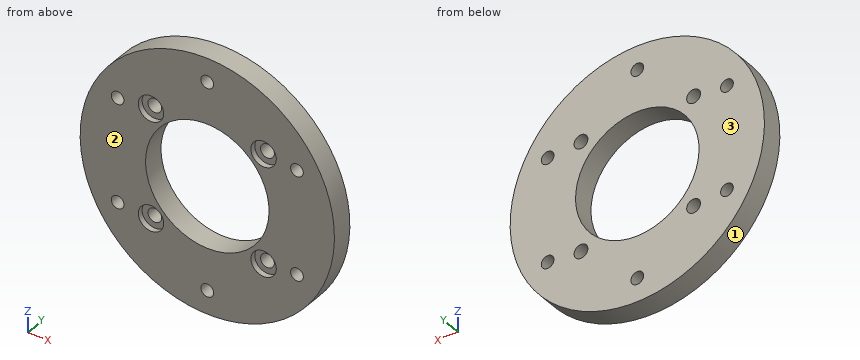
from build123d import *

# Parameters (mm, degrees)
SKETCH_1_R               = 35
EXTRUDE_1_DEPTH          = 6
HOLE_WIZARD_1_D          = 3.5
PATTERN_CIRCULAR_1_COUNT = 6
HOLE_WIZARD_2_D          = 3.8
SKETCH_8_R               = 11
CUT_EXTRUDE_1_DEPTH      = 10
HOLE_WIZARD_3_D          = 7
HOLE_WIZARD_3_DEPTH      = 1.5
SKETCH_13_R              = 17
CUT_EXTRUDE_2_DEPTH      = 10


with BuildPart() as part:
    # 草图1 → 凸台-拉伸1 (new body)
    with BuildSketch(Plane(origin=(0, 0, 0), x_dir=(1, 0, 0), z_dir=(0, 1, 0))):
        with Locations(Location((0, 0, 0), (0, 0, 270))):
            Circle(SKETCH_1_R)
    extrude(amount=EXTRUDE_1_DEPTH)

    # 孔1 (through all)
    with Locations(Plane(origin=(0, 6, 0), x_dir=(1, 0, 0), z_dir=(0, 1, 0))):
        with Locations((0, 28.5)):
            hole_wizard_1 = Hole(HOLE_WIZARD_1_D / 2)

    # 阵列(圆周)1: 孔1 ×6 about axis
    pattern_circular_1_axis = Axis((0, 0, 0), (0, 1, 0))
    for i in range(1, PATTERN_CIRCULAR_1_COUNT):
        add(hole_wizard_1.rotate(pattern_circular_1_axis, i * 360 / PATTERN_CIRCULAR_1_COUNT), mode=Mode.SUBTRACT)

    # 孔2 (through all)
    with Locations(Plane(origin=(0, 6, 0), x_dir=(1, 0, 0), z_dir=(0, 1, 0))):
        with Locations((-15.5, 15), (15.5, 15), (15.5, -15), (-15.5, -15)):
            Hole(HOLE_WIZARD_2_D / 2)

    # 草图8 → 切除-拉伸1 (cut)
    with BuildSketch(Plane(origin=(0, 6, 0), x_dir=(1, 0, 0), z_dir=(0, 1, 0))):
        with Locations(Location((0, 0, 0), (0, 0, 270))):
            Circle(SKETCH_8_R)
    extrude(amount=-CUT_EXTRUDE_1_DEPTH, mode=Mode.SUBTRACT)

    # 孔3
    with Locations(Plane(origin=(0, 0, 0), x_dir=(-1, 0, 0), z_dir=(0, -1, 0))):
        with Locations((-15.5, 15), (15.5, 15), (15.5, -15), (-15.5, -15)):
            Hole(HOLE_WIZARD_3_D / 2, depth=HOLE_WIZARD_3_DEPTH)

    # 草图13 → 切除-拉伸2 (cut)
    with BuildSketch(Plane.XZ):
        with Locations(Location((0, 0, 0), (0, 0, 270))):
            Circle(SKETCH_13_R)
    extrude(amount=-CUT_EXTRUDE_2_DEPTH, mode=Mode.SUBTRACT)


solid = part.part
CAD build for the part. Positions are in the model's coordinates, mm. Face numbers are marked on the shaded views. Coordinates: 2 decimals unless noted, no trailing zeros. Write each loop counter-clockwise with the first axis right and the second up, starting at its lowest first coordinate (ties: lowest second). Pieces come first, ordered by that corner, then holes. Notation, with made-up numbers: M -28.5,-2.5 L 29.5,-2.5 A28 cw 29.5,18.5 Z; hole C 51,-30.75 d11. An arc over 180 degrees is marked long. Answer as a JSON object with one key per item and string values. Group by question number.
1) Saw through at D-D (x = 15.5). Write the cut outline in (y, z), plus the area to 3 significant figures.
2) Mould opens along Y. For the marked faces 1, 2 and 3 say: +Y half, -Y half, draft (parallel to the pull), parting line (faces both ways), or undercut.
3) Saw through at A-A (x = 0). Write the cut outline in (y, z), plus the area to 3 significant figures.
4) Pin check, flat tips, straight feed: pin 1 Ø1.5 at (x, y) = (20, 3) entering from -Z; pin 2 Ø1 at (x, y) = (-25.5, 4) entering from +Z; pin 3 Ø1.5 at (x, y) = (-25, 3) entering from -Z. Stop position of each tip, or through.
5) Saw through at B-B (z = 4). Write the cut outline in (x, y), plus the area to 3 significant figures.
6) Saw through at C-C (y = 2.4). Give the number of separate pieces and of enclosed holes in the cut face, plus the area to 3 significant figures.
7) Wall check: line 1 (Z direction, x = 13, y = 1.05); line 2 (Z direction, x = -24.5, y = 1.5) (3 decimals); line 3 (X direction, y = 1.2, z = 15). Give the ranges that are in metal, low to high. Write a range as from..to.
Values follow:
{
 "1": {"outline": "M 0,-31.38 L 6,-31.38 L 6,-16.9 L 1.5,-16.9 L 1.5,-18.5 L 0,-18.5 Z; M 0,-11.5 L 1.5,-11.5 L 1.5,-13.1 L 6,-13.1 L 6,-6.98 L 0,-6.98 Z; M 0,6.98 L 6,6.98 L 6,13.1 L 1.5,13.1 L 1.5,11.5 L 0,11.5 Z; M 0,18.5 L 1.5,18.5 L 1.5,16.9 L 6,16.9 L 6,31.38 L 0,31.38 Z", "area": "238 mm2"},
 "2": {"face 1": "draft", "face 2": "-Y half", "face 3": "+Y half"},
 "3": {"outline": "M 0,-35 L 6,-35 L 6,-30.25 L 0,-30.25 Z; M 0,-26.75 L 6,-26.75 L 6,-17 L 0,-17 Z; M 0,17 L 6,17 L 6,26.75 L 0,26.75 Z; M 0,30.25 L 6,30.25 L 6,35 L 0,35 Z", "area": "174 mm2"},
 "4": {"pin 1": "stops at z = -29.23", "pin 2": "stops at z = 24.49", "pin 3": "stops at z = -25.24"},
 "5": {"outline": "M -34.77,0 L -16.52,0 L -16.52,6 L -34.77,6 Z; M 16.52,0 L 34.77,0 L 34.77,6 L 16.52,6 Z", "area": "219 mm2"},
 "6": {"separate pieces": "1", "enclosed holes": "11", "area": "2,840 mm2"},
 "7": {"line 1": "z = -32.5..-17.45, -12.55..-10.95, 10.95..12.55, 17.45..32.5", "line 2": "z = -24.995..-15.991, -12.509..12.509, 15.991..24.995", "line 3": "x = -31.62..-26.26, -23.1..-19, -12..-8, 8..12, 19..23.1, 26.26..31.62"}
}
